Source: three-view drawing plus pictorial views. Frame: mm from the lowest corner of the part. Coordinates: 2 decimals unless noted, no trailing zeros. Loops run counter-clockwise (first coordinate to the right, second up) from the corner with the lowest first, then second, coordinate; pieces in that order, holes last.
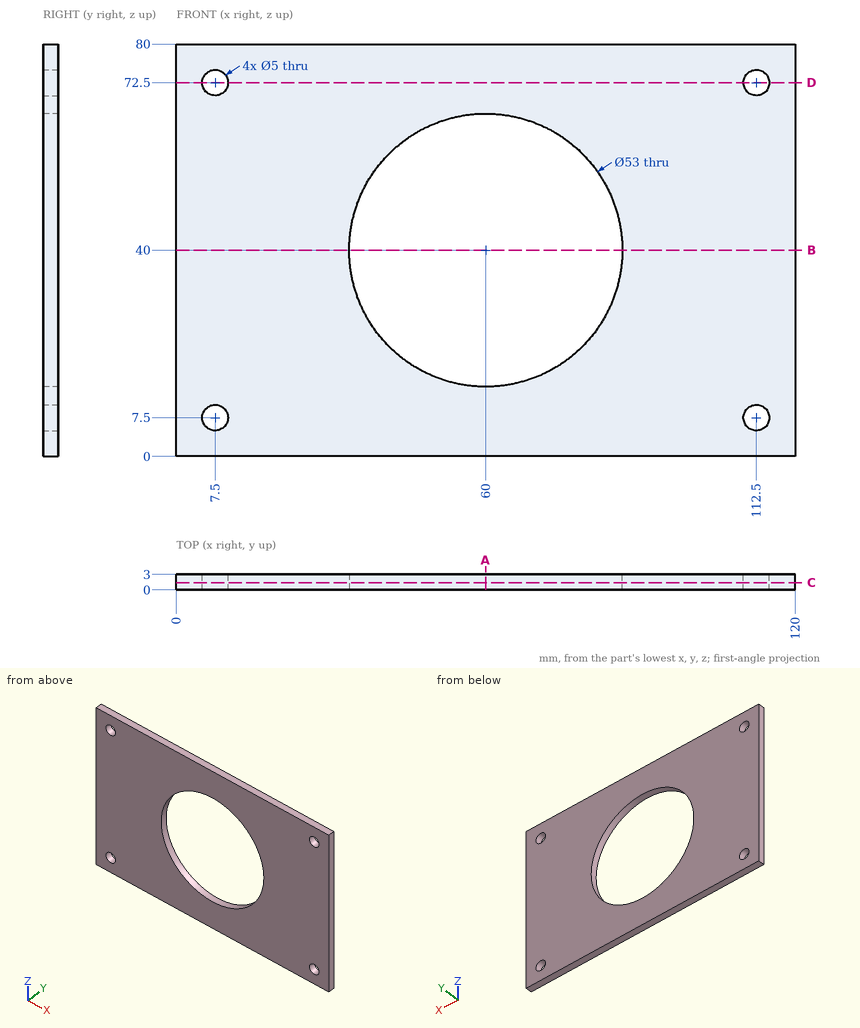
Q1. Section query B-B on z = 40. Return the cut outline in (x, y).
Q2. Material intervals for line 1 along X through (y, z) = (1.6, 7.5); line 2 along Z through (x, y) = (61, 0.3); line 3 along X through (y, z) = (1.6, 72), sorted ascending.
Q3. Section query D-D on z = 72.5. Return the cut outline in (x, y).
Q4. Section query A-A on x = 60. Return the cut outline in (y, z).
Q5. Section query C-C on y = 1.4. Return the cut outline in (x, z), then the cut area to 3 significant figures.
Q6. First-contact query: pin 1 Ø3 at (x, z) = (7.5, 7.5) entering from +Y. Flat tip, straight axial feed; report the tip coordinate or a pass-through.
Resolved:
1. outline: (0, 0) - (33.5, 0) - (33.5, 3) - (0, 3) - close; (86.5, 0) - (120, 0) - (120, 3) - (86.5, 3) - close
2. line 1: x = 0 to 5, 10 to 110, 115 to 120
2. line 2: z = 0 to 13.52, 66.48 to 80
2. line 3: x = 0 to 5.05, 9.95 to 110.05, 114.95 to 120
3. outline: (0, 0) - (5, 0) - (5, 3) - (0, 3) - close; (10, 0) - (110, 0) - (110, 3) - (10, 3) - close; (115, 0) - (120, 0) - (120, 3) - (115, 3) - close
4. outline: (0, 0) - (3, 0) - (3, 13.5) - (0, 13.5) - close; (0, 66.5) - (3, 66.5) - (3, 80) - (0, 80) - close
5. outline: (0, 0) - (120, 0) - (120, 80) - (0, 80) - close; hole circle Ø5 at (7.5, 7.5); hole circle Ø5 at (7.5, 72.5); hole circle Ø53 at (60, 40); hole circle Ø5 at (112.5, 7.5); hole circle Ø5 at (112.5, 72.5)
5. area: 7,320 mm2
6. pin 1: passes through
